Can you work these out from the model? Positions are in its coordinate system, mm. A direction names the side the tool comes from. Round coordinates to 2 decimals unless told otherwise and drop trailing zeros. Write item = value, one per line.
from build123d import *

# Parameters (mm, degrees)
SKETCH1_W           = 187.3
SKETCH1_H           = 187.3
BOSS_EXTRUDE1_DEPTH = 6.35
SKETCH2_W           = 22.55
SKETCH2_H           = 11.95
CUT_EXTRUDE1_DEPTH  = 6.35
SKETCH3_R           = 1.5
CUT_EXTRUDE2_DEPTH  = 7.35
CUT_EXTRUDE3_DEPTH  = 7.35


with BuildPart() as part:
    # Sketch1 → Boss-Extrude1 (new body)
    with BuildSketch(Plane(origin=(0, 0, 0), x_dir=(0, 0, -1), z_dir=(1, 0, 0))):
        Rectangle(SKETCH1_W, SKETCH1_H)
    extrude(amount=BOSS_EXTRUDE1_DEPTH)

    # Sketch2 → Cut-Extrude1 (cut)
    with BuildSketch(Plane(origin=(6.35, 0, 0), x_dir=(0, 0, -1), z_dir=(1, 0, 0))):
        with Locations((-70.783988916, 0)):
            Rectangle(SKETCH2_W, SKETCH2_H)
    extrude(amount=-CUT_EXTRUDE1_DEPTH, mode=Mode.SUBTRACT)

    # Sketch3 → Cut-Extrude2 (cut, through all)
    with BuildSketch(Plane(origin=(6.35, 0, 0), x_dir=(0, 0, -1), z_dir=(1, 0, 0))):
        with Locations((-66.978988916, 11)):
            Circle(SKETCH3_R)
        with Locations((-66.978988916, -11)):
            Circle(SKETCH3_R)
    extrude(amount=-CUT_EXTRUDE2_DEPTH, mode=Mode.SUBTRACT)

    # Sketch4 → Cut-Extrude3 (cut, through all)
    with BuildSketch(Plane(origin=(6.35, 0, 0), x_dir=(0, 0, -1), z_dir=(1, 0, 0))):
        Polygon((-93.65, 66.5), (-89.65, 66.5), (-89.65, 67.71), (-87.3, 67.71), (-87.3, 66.5), (-85.3, 66.5), (-85.3, 63.5), (-87.3, 63.5), (-87.3, 62.29), (-89.65, 62.29), (-89.65, 63.5), (-93.65, 63.5), align=None)
        Polygon((-87.3, -63.5), (-87.3, -62.29), (-89.65, -62.29), (-89.65, -63.5), (-93.65, -63.5), (-93.65, -66.5), (-89.65, -66.5), (-89.65, -67.71), (-87.3, -67.71), (-87.3, -66.5), (-85.3, -66.5), (-85.3, -63.5), align=None)
        Polygon((93.65, -66.5), (89.65, -66.5), (89.65, -67.71), (87.3, -67.71), (87.3, -66.5), (85.3, -66.5), (85.3, -63.5), (87.3, -63.5), (87.3, -62.29), (89.65, -62.29), (89.65, -63.5), (93.65, -63.5), align=None)
        Polygon((87.3, 63.5), (87.3, 62.29), (89.65, 62.29), (89.65, 63.5), (93.65, 63.5), (93.65, 66.5), (89.65, 66.5), (89.65, 67.71), (87.3, 67.71), (87.3, 66.5), (85.3, 66.5), (85.3, 63.5), align=None)
        Polygon((-1.5, 93.65), (-1.5, 89.65), (-2.71, 89.65), (-2.71, 87.3), (-1.5, 87.3), (-1.5, 85.3), (1.5, 85.3), (1.5, 87.3), (2.71, 87.3), (2.71, 89.65), (1.5, 89.65), (1.5, 93.65), align=None)
        Polygon((-2.71, -87.3), (-1.5, -87.3), (-1.5, -85.3), (1.5, -85.3), (1.5, -87.3), (2.71, -87.3), (2.71, -89.65), (1.5, -89.65), (1.5, -93.65), (-1.5, -93.65), (-1.5, -89.65), (-2.71, -89.65), align=None)
    extrude(amount=-CUT_EXTRUDE3_DEPTH, mode=Mode.SUBTRACT)


solid = part.part
1. For faces 1 (the flat face through (3, -63.5, 92)), 2 (the flat face through (0, 1, 1)), 3 (the flat face through (3, 80, -93.65)), 4 (the flat face through (3, -5.975, 71)), 5 (the flat face through (3, -63.5, -92)), which set-ups out of +Z, -Z, +X, -X, +Y, -Y let a thin tool reach every point of the face, with its end or its side?
Entries:
face_1 = +Z, +X, -X
face_2 = +Z, -Z, -X, +Y, -Y
face_3 = -Z, +X, -X, +Y, -Y
face_4 = +X, -X
face_5 = -Z, +X, -X
2. We'd pull the mould along Y, two halves only. Please class faces 6 (the flat face through (3, -93.65, -47)), 7 (the flat face through (3, 5.975, 71)), 8 (the flat face through (6.35, 1, 1)): released by +Y, released by -Y, zero draft, split by the parting line, or undercut.
Entries:
face_6 = released by -Y
face_7 = undercut
face_8 = zero draft
3. I need wall thicknesses on line 1 (Z direction, x = 2.75, y = -5); line 2 (Y direction, x = 2.25, z = 61) (3 decimals); line 3 (Z direction, x = 2, y = -10). Which ranges of each line are inside material? Lowest first, please. Write a range as [from, to].
Entries:
line_1 = [-93.65, 59.51], [82.06, 93.65]
line_2 = [-93.65, -5.975], [5.975, 93.65]
line_3 = [-93.65, 65.86], [68.1, 93.65]
